from build123d import *

# Parameters (mm, degrees)
SKETCH_1_R                   = 13.5
EXTRUDE_7_DEPTH              = 27
EXTRUDE_9_DEPTH              = 13.5
EXTRUDE_10_DEPTH             = 13.5
EXTRUDE_START                = -27
SKETCH_9_R                   = 12
EXTRUDE_11_DEPTH             = 4
EXTRUDE_START_2              = -31
SKETCH_10_R                  = 13.5
EXTRUDE_12_DEPTH             = 17
EXTRUDE_START_3              = -48
SKETCH_11_R                  = 4
EXTRUDE_13_DEPTH             = 5
EXTRUDE_START_4              = -53
SKETCH_12_R                  = 2
EXTRUDE_14_DEPTH             = 1
HOLE_WIZARD_M3_1_D           = 3.6
HOLE_WIZARD_M3_1_ON_FACE_2_D = 3.6


with BuildPart() as part:
    # ｽｹｯﾁ1 → ﾎﾞｽ - 押し出し7 (new body)
    with BuildSketch(Plane(origin=(0, 0, 0), x_dir=(1, 0, 0), z_dir=(0, 1, 0))):
        Circle(SKETCH_1_R)
        with BuildLine():
            Line((-13.5, -13.5), (0, -13.5))
            ThreePointArc((0, -13.5), (-9.545941546, -9.545941546), (-13.5, 0))
            Line((-13.5, 0), (-13.5, -13.5))
        make_face()
        with BuildLine():
            ThreePointArc((13.5, 0), (9.545941546, -9.545941546), (0, -13.5))
            Line((0, -13.5), (13.5, -13.5))
            Line((13.5, -13.5), (13.5, 0))
        make_face()
        Polygon((20, -13.5), (20, -14.5), (-20, -14.5), (-20, -13.5), (0, -13.5), align=None)
    extrude(amount=EXTRUDE_7_DEPTH)

    # ｽｹｯﾁ2 → ﾎﾞｽ - 押し出し9 (add)
    with BuildSketch(Plane(origin=(0, 0, 13.5), x_dir=(-1, 0, 0), z_dir=(0, 0, -1))):
        with BuildLine():
            Line((13.5, 10.575), (16.75, 10.575))
            ThreePointArc((16.75, 10.575), (19.675, 13.5), (16.75, 16.425))
            Line((16.75, 16.425), (13.5, 16.425))
            Line((13.5, 16.425), (13.5, 10.575))
        make_face()
    extrude(amount=EXTRUDE_9_DEPTH)

    # ｽｹｯﾁ3 → ﾎﾞｽ - 押し出し10 (add)
    with BuildSketch(Plane(origin=(0, 0, 13.5), x_dir=(-1, 0, 0), z_dir=(0, 0, -1))):
        with BuildLine():
            Line((-13.5, 16.425), (-16.75, 16.425))
            ThreePointArc((-16.75, 16.425), (-19.675, 13.5), (-16.75, 10.575))
            Line((-16.75, 10.575), (-13.5, 10.575))
            Line((-13.5, 10.575), (-13.5, 16.425))
        make_face()
    extrude(amount=EXTRUDE_10_DEPTH)

    # ｽｹｯﾁ9 → ﾎﾞｽ - 押し出し11 (add)
    with BuildSketch(Plane.XZ.offset(EXTRUDE_START)):
        with Locations(Location((0, 0, 0), (0, 0, 270))):
            Circle(SKETCH_9_R)
    extrude(amount=-EXTRUDE_11_DEPTH)

    # ｽｹｯﾁ10 → ﾎﾞｽ - 押し出し12 (add)
    with BuildSketch(Plane.XZ.offset(EXTRUDE_START_2)):
        with Locations(Location((0, 0, 0), (0, 0, 270))):
            Circle(SKETCH_10_R)
    extrude(amount=-EXTRUDE_12_DEPTH)

    # ｽｹｯﾁ11 → ﾎﾞｽ - 押し出し13 (add)
    with BuildSketch(Plane.XZ.offset(EXTRUDE_START_3)):
        with Locations(Location((0, 0, 0), (0, 0, 270))):
            Circle(SKETCH_11_R)
    extrude(amount=-EXTRUDE_13_DEPTH)

    # ｽｹｯﾁ12 → ﾎﾞｽ - 押し出し14 (add)
    with BuildSketch(Plane.XZ.offset(EXTRUDE_START_4)):
        with Locations(Location((0, 0, 0), (0, 0, 270))):
            Circle(SKETCH_12_R)
    extrude(amount=-EXTRUDE_14_DEPTH)

    # M3 すきま穴1 (through all)
    with Locations(Plane(origin=(16.75, 21, 13.5), x_dir=(-1, 0, 0), z_dir=(0, 0, -1))):
        with Locations((0, 0), (0, -15), (33.5, 0), (33.5, -15)):
            Hole(HOLE_WIZARD_M3_1_D / 2)

    # M3 すきま穴1 on face 2 (through all)
    with Locations(Plane(origin=(16.75, 13.5, 0), x_dir=(-1, 0, 0), z_dir=(0, 0, -1))):
        with Locations((0, 0), (33.5, 0)):
            Hole(HOLE_WIZARD_M3_1_ON_FACE_2_D / 2)


solid = part.part
Geometry: final body of the model. Coordinates: model frame, mm. A direction names the side the tool comes from. Round coordinates to 2 decimals unless told otherwise and drop trailing zeros. Loops run counter-clockwise (first coordinate to the right, second up) from the corner with the lowest first, then second, coordinate; pieces in that order, holes last. Notation, with made-up numbers: (57.25, 64) -> (102.25, 64) arc R27 cw to (102.25, 101) -> close; hole circle Ø10 at (87, -17). An arc over 180 degrees is marked (long way). One line per question, with ' | ' between items. Start each with the question number.
1. Set-up query: faces 1 (the face through (-15, 16.425, 7)), 2 (the face through (15, 16.425, 7)), 3 (the face through (-3.905, 50.465, 0.867)). Return all of +Z, -Z, +X, -X, +Y, -Y with unobstructed straight access to the full face (end or side cutting, diameter ignored); none if empty.
2. Contact query for flat-ended pins moving along their axis: pin 1 (5 mm diameter, centred on x = 13, z = -6.5, fed in from +Y); pin 2 (14 mm diameter, centred on x = 7, z = -5.5, fed in from +Y); pin 3 (3.5 mm diameter, centred on x = 14.5, z = 5, fed in from +Y); pin 4 (5 mm diameter, centred on x = 16.5, y = 14.5, fed in from -Z). Output: stop coordinate, or through.
3. Mould query, pull axis Y, two halves, no side actions, for faces 4 (the face through (-15, 15, 0)), 5 (the face through (-2, 31, 12)), 6 (the face through (-1, 53, 2)), 7 (the face through (16.516, 15.285, 7.352)). Classes: pulls with the +Y half, pulls with the -Y half, needs draft (parallel to the pull), parting line crosses it, or undercut.
4. Section B-B on z = 10.75. Output: boundary loops of the cut face in (x, y) (3 decimals).
5. Section C-C on x = 5. Output: boundary loops of the cut face in (y, z), and give its area (3 significant figures).
6. Section D-D on y = 13.5. Output: boundary loops of the cut face in (x, z) (3 decimals).
7. Section A-A on y = 6. Output: boundary loops of the cut face in (x, z), and give its area (3 significant figures).
8. Line query: line 1 along Y through (x, z) = (16.75, 13.85); line 2 along Y through (x, z) = (-16.75, 4.5) (3 decimals); line 3 along Y through (x, z) = (-6.5, 10.5). Output: solid intervals per line, ascending. Write a range as [from, to].
Returned:
1) face 1: -Z, -X, +Y | face 2: -Z, +X, +Y | face 3: +Y
2) pin 1: stops at y = 48 | pin 2: stops at y = 54 | pin 3: stops at y = 27 | pin 4: stops at z = 0
3) face 4: needs draft | face 5: undercut | face 6: pulls with the +Y half | face 7: undercut
4) outline: (-16.75, 10.575) -> (-13.5, 10.575) -> (-13.5, 0) -> (13.5, 0) -> (13.5, 10.575) -> (16.75, 10.575) arc R2.925 ccw to (16.75, 16.425) -> (13.5, 16.425) -> (13.5, 27) -> (5.333, 27) -> (5.333, 31) -> (8.166, 31) -> (8.166, 48) -> (-8.166, 48) -> (-8.166, 31) -> (-5.333, 31) -> (-5.333, 27) -> (-13.5, 27) -> (-13.5, 16.425) -> (-16.75, 16.425) arc R2.925 ccw to start; hole circle Ø3.6 at (-16.75, 13.5); hole circle Ø3.6 at (16.75, 13.5)
5) outline: (0, -12.54) -> (27, -12.54) -> (27, -10.91) -> (31, -10.91) -> (31, -12.54) -> (48, -12.54) -> (48, 12.54) -> (31, 12.54) -> (31, 10.91) -> (27, 10.91) -> (27, 14.5) -> (0, 14.5) -> close | area: 1,240 mm2
6) outline: (-20, 13.5) -> (-19.675, 13.5) -> (-19.675, 0) -> (-18.55, 0) -> (-18.55, 14.5) -> (-20, 14.5) -> close; (-14.95, 0) -> (-13.5, 0) arc R13.5 ccw to (13.5, 0) -> (14.95, 0) -> (14.95, 14.5) -> (-14.95, 14.5) -> close; (18.55, 0) -> (19.675, 0) -> (19.675, 13.5) -> (20, 13.5) -> (20, 14.5) -> (18.55, 14.5) -> close
7) outline: (-20, 13.5) -> (-18.55, 13.5) -> (-18.55, 14.5) -> (-20, 14.5) -> close; (-14.95, 13.5) -> (-13.5, 13.5) -> (-13.5, 0) arc R13.5 ccw to (13.5, 0) -> (13.5, 13.5) -> (14.95, 13.5) -> (14.95, 14.5) -> (-14.95, 14.5) -> close; (18.55, 13.5) -> (20, 13.5) -> (20, 14.5) -> (18.55, 14.5) -> close | area: 684 mm2
8) line 1: y = [0, 4.2], [7.8, 11.7], [15.3, 19.2], [22.8, 27] | line 2: y = [10.575, 11.7], [15.3, 16.425] | line 3: y = [0, 27], [31, 48]
